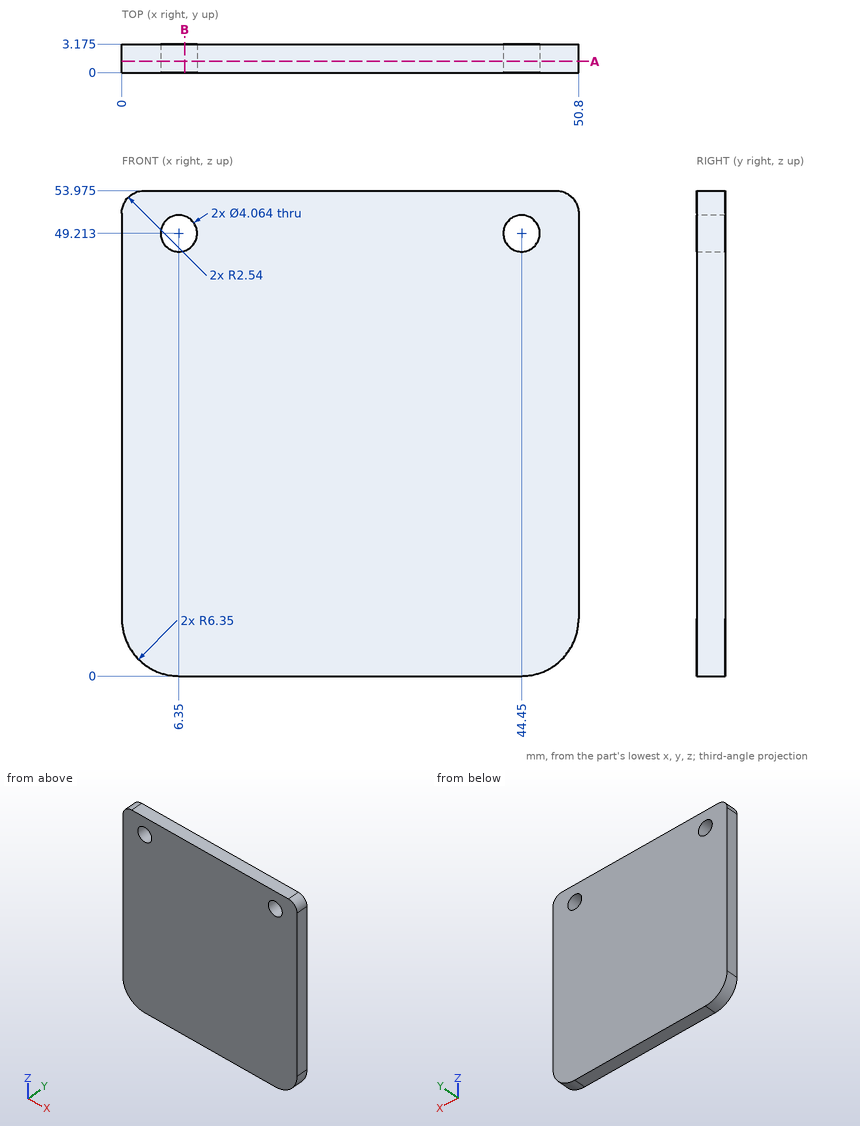
Source: three-view drawing plus pictorial views. Frame: mm from the lowest corner of the part. Coordinates: 2 decimals unless noted, no trailing zeros. Loops run counter-clockwise (first coordinate to the right, second up) from the corner with the lowest first, then second, coordinate; pieces in that order, holes last. Notation, with made-up numbers: (8.5, -24) -> (44.5, -24) arc R22 cw to (44.5, 1) -> close; hole circle Ø4 at (-40, -15.75). An arc over 180 degrees is marked (long way). One line per item, written item: value.
(1) Cut plane A-A (y = 1.25). Give the number of separate pieces and of enclosed holes in the cut face, then the cut area to 3 significant figures.
Answer below:
separate pieces: 1
enclosed holes: 2
area: 2,700 mm2
(2) Ray query, line 1 along Z through (x, y) = (44.45, 1.8) (1 decimal); line 2 along X through (y, z) = (3, 50.5); line 3 along X through (y, z) = (2.5, 50) (1 decimal). Return the intervals inside material, ascending.
Answer below:
line 1: z = 0 to 47.2, 51.2 to 54
line 2: x = 0 to 4.78, 7.92 to 42.88, 46.02 to 50.8
line 3: x = 0 to 4.5, 8.2 to 42.6, 46.3 to 50.8
(3) Cut plane B-B (x = 7). Output: boundary loops of the cut face in (y, z) (1 decimal), then the cut area to 3 significant figures.
Answer below:
outline: (0, 0) -> (3.2, 0) -> (3.2, 47.3) -> (0, 47.3) -> close; (0, 51.1) -> (3.2, 51.1) -> (3.2, 54) -> (0, 54) -> close
area: 159 mm2
(4) Pin query (flat end, axial travel): pin 1 Ø3.5 at (x, z) = (44.45, 49.21) entering from +Y; pin 2 Ø6.5 at (x, z) = (6.35, 49.21) entering from +Y (1 decimal). Return the tip coordinate at first contact, or that it passes through.
Answer below:
pin 1: passes through
pin 2: stops at y = 3.2
